Print and shaded views of the part. All mm, measured from the part's lowest x, y and z. A direction names the side the tool comes from. Coordinates: 2 decimals unless noted, no trailing zeros. Order: outer loops, then holes, each group sorted by start corner. A loop starts at its lowest first (then second) coordinate and runs counter-clockwise, first axis right, second up. Notation, with made-up numbers: (76.5, 7) -> (90.5, 7) arc R29 cw to (90.5, 33) -> close; hole circle Ø9 at (-38, 71). An arc over 180 degrees is marked (long way). Return JSON: item names as keys, results as strings. Group by question number.
1) Probe line 1 (Y direction, x = 40.75, z = 150); line 2 (Z direction, x = 25, y = 9.75). List the from-to ranges inside material, lowest first.
2) Pull direction Y, two halves, no side cores. Call the marked faces 4, 5, 6 and 7: +Y half, -Y half, draft (parallel to the pull), parting line (faces both ways), or undercut.
3) Cut at B-B (y = 29.5). Write the cut outline in (x, z), and give its area (3 significant figures).
4) Cut at C-C (z = 143). Write the cut outline in (x, y).
5) Flat gauge pins, fed straight in: pin 1 (1 mm diameter, centred on x = 43.5, y = 6, fed in from +Z) (1 decimal); pin 2 (16 mm diameter, centred on x = 26.5, y = 18.5, fed in from +Z); pin 3 (6 mm diameter, centred on x = 35, y = 24, fed in from -Z). Where does each tip first touch, or does it go through?
6) Which spindle directions (+Z, -Z, +X, -X, +Y, -Y) get a long thin tool onto all of the face, cutting with end or side? Do the marked faces 1, 2 and 3. Say none if no direction does.
7) Cut at A-A (x = 29.5). Write the cut outline in (y, z).
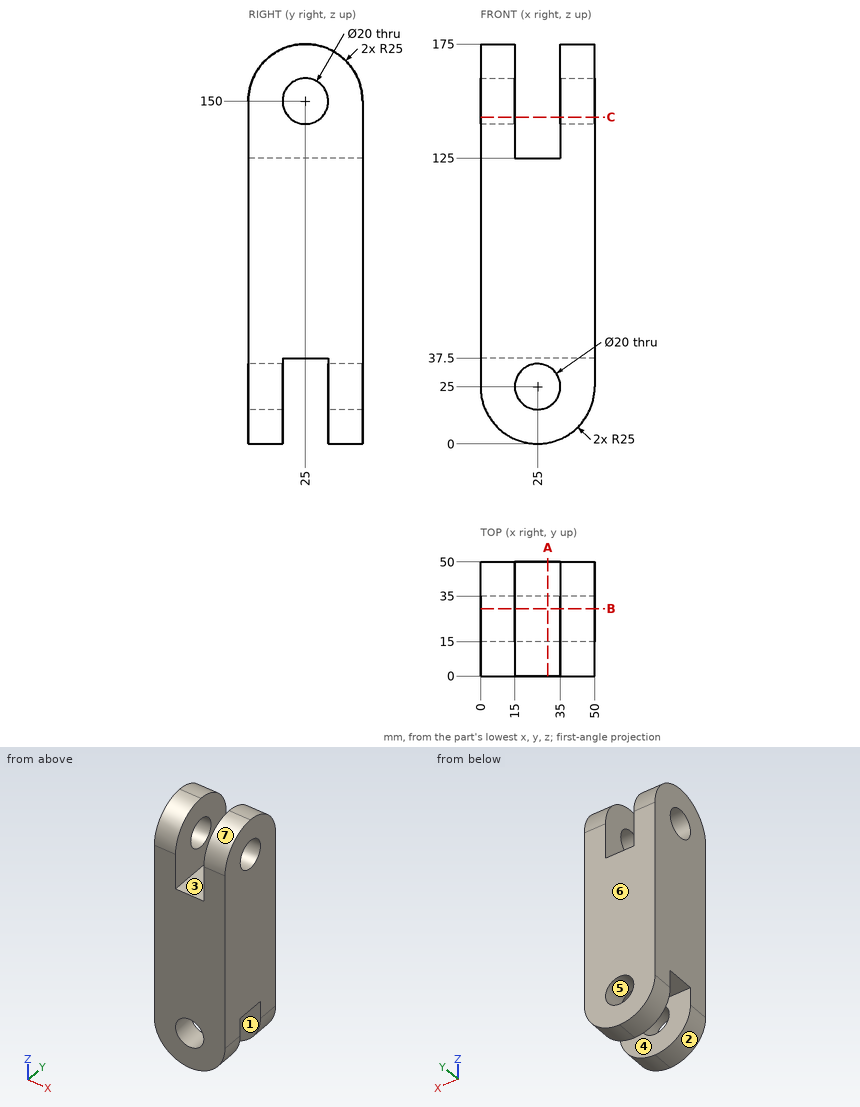
Answers below:
{
 "1": {"line 1": "y = 0 to 15, 35 to 50", "line 2": "z = 0 to 15, 35 to 125"},
 "2": {"face 4": "undercut", "face 5": "draft", "face 6": "+Y half", "face 7": "-Y half"},
 "3": {"outline": "(0, 37.5) -> (50, 37.5) -> (50, 141.07) -> (35, 141.07) -> (35, 125) -> (15, 125) -> (15, 141.07) -> (0, 141.07) -> close; (0, 158.93) -> (15, 158.93) -> (15, 174.59) -> (0, 174.59) -> close; (35, 158.93) -> (50, 158.93) -> (50, 174.59) -> (35, 174.59) -> close", "area": "5,330 mm^2"},
 "4": {"outline": "(0, 0) -> (15, 0) -> (15, 17.86) -> (0, 17.86) -> close; (0, 32.14) -> (15, 32.14) -> (15, 50) -> (0, 50) -> close; (35, 0) -> (50, 0) -> (50, 17.86) -> (35, 17.86) -> close; (35, 32.14) -> (50, 32.14) -> (50, 50) -> (35, 50) -> close"},
 "5": {"pin 1": "stops at z = 166.8", "pin 2": "stops at z = 125", "pin 3": "stops at z = 37.5"},
 "6": {"face 1": "-Z, +X, -X", "face 2": "-Z, -X, +Y, -Y", "face 3": "+Z, +Y, -Y"},
 "7": {"outline": "(0, 0.41) -> (15, 0.41) -> (15, 16.07) -> (0, 16.07) -> close; (0, 33.93) -> (15, 33.93) -> (15, 37.5) -> (35, 37.5) -> (35, 33.93) -> (50, 33.93) -> (50, 125) -> (0, 125) -> close; (35, 0.41) -> (50, 0.41) -> (50, 16.07) -> (35, 16.07) -> close"}
}
